Part model, mm, in its own coordinate system. A direction names the side the tool comes from. Round coordinates to 2 decimals unless told otherwise and drop trailing zeros. Write each loop counter-clockwise with the first axis right and the second up, starting at its lowest first coordinate (ties: lowest second). Pieces come first, ordered by that corner, then holes.
1) Saw through at A-A on x = 10.25. Write the cut outline in (y, z) (3 decimals), and give its area (3 significant figures).
2) Drill centre lines: L1, parallel to X at y = 1.5, z = 3.5; L2, parallel to Z at x = 6.75, y = 1.5; L3, parallel to Z at x = 11.5, y = 12.25. Where is each one in solid material? Low to high.
3) Pull direction Z, two halves, no side cores. Call faces 1 (the cylindrical face through (5.21, 7.83, 9.1)), 2 (the flat face through (8, 8, -15)), 3 (the flat face through (3, 15.875, 0)), 4 (the flat face through (10.677, 7.826, -10.735)): +Z half, -Z half, draft (parallel to the pull), parting line (faces both ways), or undercut.
4) Saw through at D-D on z = -4.75. Write the cut outline in (x, y) (3 decimals), and give its area (3 significant figures).
5) Saw through at C-C on x = 8.75. Write the cut outline in (y, z) (3 decimals).
6) Saw through at B-B on y = 9.75. Write the cut outline in (x, z), and give its area (3 significant figures).
7) Flat gauge pin, fed straight in: pin 1 (9.5 mm diameter, centred on y = 9, z = 1, fed in from +X). Where does the tip first touch, or does it go through?
8) Which spindle directions (+Z, -Z, +X, -X, +Y, -Y) get a long thin tool onto all of the face, cutting with end or side? Do faces 5 (the flat face through (7, 8, 15)), 6 (the flat face through (4, 8, 0)). Say none if no direction does.
Solid Edge part; units mm, degrees
sketch "Sketch1" plane through (0, 0, 0) normal (0, -1, 0) x (1, 0, 0)
  line L0 (15, -15) -> (0, -15)
  line L1 (0, 15) -> (0, -15)
  line L2 (0, 15) -> (15, 15)
  line L3 (15, 15) -> (15, 12.9464)
  arc A0 (13.1743, 10.954) -> (15, 12.9464) centre (13, 12.9464) ccw
  line L4 (13.1743, 10.954) -> (8.1078, 10.5107)
  arc A1 (8.1078, 10.5107) -> (4, 6.0279) centre (8.5, 6.0279) ccw
  line L5 (4, -6.0279) -> (4, 6.0279)
  arc A2 (4, -6.0279) -> (8.1078, -10.5107) centre (8.5, -6.0279) ccw
  line L6 (13.1743, -10.954) -> (8.1078, -10.5107)
  arc A3 (13.1743, -10.954) -> (15, -12.9464) centre (13, -12.9464) cw
  line L7 (15, -15) -> (15, -12.9464)
  dimension "D1" = 15
extrude "Protrusion1" add sketch "Sketch1" against normal blind 15.875
Completed:
1. outline: (0, -15) - (15.875, -15) - (15.875, -10.698) - (0, -10.698) - close; (0, 10.698) - (15.875, 10.698) - (15.875, 15) - (0, 15) - close
1. area: 137 mm2
2. L1: x = 0 to 4
2. L2: z = -15 to -10.17, 10.17 to 15
2. L3: z = -15 to -10.81, 10.81 to 15
3. face 1: undercut
3. face 2: -Z half
3. face 3: draft
3. face 4: undercut
4. outline: (0, 0) - (4, 0) - (4, 15.875) - (0, 15.875) - close
4. area: 63.5 mm2
5. outline: (0, -15) - (15.875, -15) - (15.875, -10.567) - (0, -10.567) - close; (0, 10.567) - (15.875, 10.567) - (15.875, 15) - (0, 15) - close
6. outline: (0, -15) - (15, -15) - (15, -12.95) arc R2 ccw to (13.17, -10.95) - (8.11, -10.51) arc R4.5 cw to (4, -6.03) - (4, 6.03) arc R4.5 cw to (8.11, 10.51) - (13.17, 10.95) arc R2 ccw to (15, 12.95) - (15, 15) - (0, 15) - close
6. area: 222 mm2
7. pin 1: stops at x = 4
8. face 5: +Z, +X, -X, +Y, -Y
8. face 6: +X, +Y, -Y
